Model file for the job. Use its own axes, mm. A direction names the side the tool comes from. Give positions to 0.01 mm unless a question says otherwise; leave off trailing zeros. Loops run counter-clockwise (first coordinate to the right, second up) from the corner with the lowest first, then second, coordinate; pieces in that order, holes last. Notation, with made-up numbers: (5.25, -18) - (54.25, -18) arc R20 ccw to (54.25, 4) - close; hole circle Ø5 at (65.25, 28.5). An arc over 180 degrees is marked (long way). Answer as CSV lines item,"result". Start each with the question number.
Item 1: Pin check, flat tips, straight feed: pin 1 (6 mm diameter, centred on y = 3, z = 31, fed in from +X); pin 2 (4.5 mm diameter, centred on x = 12.37, z = 12.37, fed in from -Y); pin 3 (5.5 mm diameter, centred on x = 0, z = -17.5, fed in from +Y); pin 4 (2 mm diameter, centred on x = -17.5, z = 0, fed in from +Y). Stop position of each tip, or through.
Item 2: Saw through at A-A on y = 7.75. State how many separate pieces and enclosed holes the cut face has, plus the area to 3 significant figures.
Item 3: Tool access for faces 4 (the flat face through (-1, -8.45, 1)), 5 (the flat face through (23.1, -9.45, 36.5)), 6 (the cylindrical face through (11.46, 7.422, -13.808)): list every direction of +Z, -Z, +X, -X, +Y, -Y with a clear straight run to the whole face (end or side of a thin tool).
Item 4: Drill centre lines: L1, parallel to Y at x = 8, z = -18; L2, parallel to Z at x = -17, y = -2.5; L3, parallel to Z at x = -25, y = -8.5. Where is each one in solid material? Low to high. Write a range as from..to.
Item 5: Pull direction Z, two halves, no side cores. Call faces 1 (the cylindrical face through (20.765, -2.055, 39.923)), 2 (the cylindrical face through (15.88, 7.42, -0.51)), 3 (the flat face through (0, 9.45, 0)): pulls with the +Z half, pulls with the -Z half, needs draft (parallel to the pull), parting line crosses it, or undercut.
Item 6: Saw through at B-B on y = -6.25. Give the cut face in (x, z).
from build123d import *

# Parameters (mm, degrees)
SKETCH2_R                = 43
CUT_EXTRUDE1_DEPTH       = 1
M3_CLEARANCE_HOLE1_D     = 3.4
M3_CLEARANCE_HOLE1_DEPTH = 4
M3_CLEARANCE_HOLE1_TIP   = 1.021463052


with BuildPart() as part:
    # Sketch1 → Revolve1 (revolve)
    with BuildSketch(Plane.XY, mode=Mode.PRIVATE) as revolve1_sk:
        Polygon((0, -9.45), (0, 9.45), (-21.5, 9.45), (-45, 5.55), (-45, -9.45), align=None)
    revolve(revolve1_sk.sketch.rotate(Axis((0, -9.45, 0), (0, 1, 0)), 180), axis=Axis((0, -9.45, 0), (0, 1, 0)))

    # Sketch2 → Cut-Extrude1 (cut)
    with BuildSketch(Plane.XZ.offset(9.45)):
        Circle(SKETCH2_R)
    extrude(amount=-CUT_EXTRUDE1_DEPTH, mode=Mode.SUBTRACT)

    # M3 Clearance Hole1
    with Locations(Plane(origin=(0, 9.45, 0), x_dir=(1, 0, 0), z_dir=(0, 1, 0))):
        with Locations((0, 17.5), (-12.374368671, 12.374368671), (-17.5, 0), (-12.374368671, -12.374368671), (0, -17.5), (12.374368671, -12.374368671), (17.5, 0), (12.374368671, 12.374368671)):
            Hole(M3_CLEARANCE_HOLE1_D / 2, depth=M3_CLEARANCE_HOLE1_DEPTH)
            with Locations((0, 0, -(M3_CLEARANCE_HOLE1_DEPTH + M3_CLEARANCE_HOLE1_TIP / 2))):  # 118° drill point
                Cone(0, M3_CLEARANCE_HOLE1_D / 2, M3_CLEARANCE_HOLE1_TIP, mode=Mode.SUBTRACT)


solid = part.part
Responses:
1,pin 1,"x = 35.23"
1,pin 2,"y = -8.45"
1,pin 3,"y = 9.45"
1,pin 4,"y = 5.03"
2,separate pieces,"1"
2,enclosed holes,"8"
2,area,"3,090 mm2"
3,face 4,"-Y"
3,face 5,"+Z, -Z, +X, -X, -Y"
3,face 6,"+Y"
4,L1,"-8.45..9.45"
4,L2,"-41.67..41.67"
4,L3,"-37.42..-34.99, 34.99..37.42"
5,face 1,"parting line crosses it"
5,face 2,"undercut"
5,face 3,"needs draft"
6,outline,"circle Ø90 at (0, 0)"
